Autodesk Inventor part; units mm, degrees
ref_plane "YZ Plane" through (0, 0, 0) normal (1, 0, 0) x (0, 1, 0)
ref_plane "XZ Plane" through (0, 0, 0) normal (0, 1, 0) x (-1, 0, 0)
ref_plane "XY Plane" through (0, 0, 0) normal (0, 0, 1) x (1, 0, 0)
sketch "Sketch1" plane through (0, 0, 0) normal (0, 0, 1) x (1, 0, 0)
  line L0 (-9.6332, 12.3072) -> (10.3668, 12.3072)
  line L1 (10.3668, 12.3072) -> (10.3668, -12.6928)
  line L2 (10.3668, -12.6928) -> (-9.6332, -12.6928)
  line L3 (-9.6332, -12.6928) -> (-9.6332, 12.3072)
  line L4 (-4.3832, -2.6928) -> (5.1168, -2.6928)
  line L5 (5.1168, -2.6928) -> (5.1168, -7.7928)
  line L6 (5.1168, -7.7928) -> (-4.3832, -7.7928)
  line L7 (-4.3832, -7.7928) -> (-4.3832, -2.6928)
  line L8 (-1.0332, -2.6928) -> (-1.0332, -7.7928)
  line L9 (1.7668, -2.6928) -> (1.7668, -7.7928)
  line L10 (-1.0332, -2.6928) -> (-1.0332, 0.3072)
  line L11 (1.7668, -2.6928) -> (1.7668, 0.3072)
  line L12 (-1.0332, 0.3072) -> (-6.6332, 12.3072)
  line L13 (1.7668, 0.3072) -> (7.3668, 12.3072)
  line L14 (-1.0332, -7.7928) -> (-1.0332, -12.6928)
  line L15 (1.7668, -7.7928) -> (1.7668, -12.6928)
  point P0 (0, 0)
  dimension "d0" = 20
  dimension "d1" = 25
  dimension "d2" = 3.35
  dimension "d3" = 3.35
  dimension "d4" = 2.8
  dimension "d5" = 5.1
  dimension "d6" = 5.25
  dimension "d7" = 9.5
  dimension "d9" = 15
  dimension "d10" = 4.9
  dimension "d11" = 3
  dimension "d12" = 3
  dimension "d13" = 3
  dimension "d14" = 3
extrude "Extrusion1" add sketch "Sketch1" along normal blind 3 contours L0 L12 L10 L4 L7 L6 L14 L2 L3 | L0 L1 L2 L15 L6 L5 L4 L11 L13
extrude "Extrusion2" add sketch "Sketch1" against normal blind 5 contours L0 L12 L10 L4 L7 L6 L14 L2 L3 | L0 L13 L11 L4 L10 L12 | L0 L1 L2 L15 L6 L5 L4 L11 L13 | L14 L6 L15 L2 | L4 L9 L6 L8
sketch "Sketch2" plane through (0, 0, -5) normal (0, 0, -1) x (-1, 0, 0)
  line L0 (-1.7668, -2.6928) -> (-1.7668, -7.7928)
  line L1 (-1.7668, -7.7928) -> (-5.1168, -7.7928)
  line L2 (-5.1168, -7.7928) -> (-5.1168, -2.6928)
  line L3 (-5.1168, -2.6928) -> (-1.7668, -2.6928)
  line L4 (1.0332, -7.7928) -> (1.0332, -2.6928)
  line L5 (1.0332, -2.6928) -> (4.3832, -2.6928)
  line L6 (4.3832, -2.6928) -> (4.3832, -7.7928)
  line L7 (4.3832, -7.7928) -> (1.0332, -7.7928)
  line L8 (9.6332, 12.3072) -> (-10.3668, 12.3072)
  line L9 (-10.3668, 12.3072) -> (-10.3668, -12.6928)
  line L10 (-10.3668, -12.6928) -> (9.6332, -12.6928)
  line L11 (9.6332, -12.6928) -> (9.6332, 12.3072)
  line L12 (1.0332, -12.6928) -> (1.0332, -7.7928)
  line L13 (-1.7668, -2.6928) -> (1.0332, -2.6928)
  line L14 (1.0332, -2.6928) -> (1.0332, -7.7928)
  line L15 (1.0332, -7.7928) -> (-1.7668, -7.7928)
  line L16 (-1.7668, -7.7928) -> (-1.7668, -2.6928)
  point P0 (0, 0)
extrude "Extrusion3" cut sketch "Sketch2" against normal blind 3.6 contours L13 L4 L15 L0
chamfer "Chamfer1" distance 12 distance2 3 1 edges at (0.3668, 12.3072, 0) measured on face at (-0.0999, 8.3072, 0)
sketch "Sketch3" plane through (0, 0, 3) normal (0, 0, 1) x (1, 0, 0)
  line L0 (-9.6332, 12.3072) -> (-9.6332, -12.6928)
  line L1 (-9.6332, -12.6928) -> (-1.0332, -12.6928)
  line L2 (-1.0332, -12.6928) -> (-1.0332, -7.7928)
  line L3 (-1.0332, -7.7928) -> (-4.3832, -7.7928)
  line L4 (-4.3832, -7.7928) -> (-4.3832, -2.6928)
  line L5 (-4.3832, -2.6928) -> (-1.0332, -2.6928)
  line L6 (-1.0332, -2.6928) -> (-1.0332, 0.3072)
  line L7 (-1.0332, 0.3072) -> (-6.6332, 12.3072)
  line L8 (-6.6332, 12.3072) -> (-9.6332, 12.3072)
  line L9 (10.3668, -12.6928) -> (10.3668, 12.3072)
  line L10 (10.3668, 12.3072) -> (7.3668, 12.3072)
  line L11 (7.3668, 12.3072) -> (1.7668, 0.3072)
  line L12 (1.7668, 0.3072) -> (1.7668, -2.6928)
  line L13 (1.7668, -2.6928) -> (5.1168, -2.6928)
  line L14 (5.1168, -2.6928) -> (5.1168, -7.7928)
  line L15 (5.1168, -7.7928) -> (1.7668, -7.7928)
  line L16 (1.7668, -7.7928) -> (1.7668, -12.6928)
  line L17 (1.7668, -12.6928) -> (10.3668, -12.6928)
  point P0 (0, 0)
  point P1 (-6.6332, 5.8072)
  point P2 (7.3668, 5.8072)
  point P3 (-6.6332, -9.6928)
  point P4 (7.3668, -9.6928)
  dimension "d24" = 25
  dimension "d25" = 6.5
  dimension "d26" = 3
  dimension "d27" = 4.9
  dimension "d28" = 3
  dimension "d29" = 3
  dimension "d37" = 5.25
  dimension "d38" = 3
  dimension "d39" = 3
hole "Hole1" at (-6.6332, 5.8072, 3) at (7.3668, 5.8072, 3) at (-6.6332, -9.6928, 3) at (7.3668, -9.6928, 3) direction (0, 0, -1) diameter 2.5 end through all
fillet "Fillet1" radius 1.5 2 edges at (-6.6332, 12.3072, 0) (7.3668, 12.3072, 0)
fillet "Fillet2" radius 2 4 edges at (-9.6332, 12.3072, -1) (10.3668, 12.3072, -1) (10.3668, -12.6928, -1) (-9.6332, -12.6928, -1)
equation "\"d3\" = d2"
equation "\"d6\" = -0.5 * d7 + 0.5 * d0"
equation "\"d12\" = d11"
equation "\"d14\" = d13"
properties part number "3DP_PLA_Part_Detector_Bottom_Half" material "ABS Plastic"
The listing builds one solid part. Answer for the finished solid, in the listing's coordinates (mm). A direction names the side the tool comes from. Coordinates: 2 decimals unless noted, no trailing zeros. Write each loop counter-clockwise with the first axis right and the second up, starting at its lowest first coordinate (ties: lowest second). Pieces come first, ordered by that corner, then holes. Notation, with made-up numbers: (53.25, 74) - (81.25, 74) arc R30 ccw to (81.25, 101) - close; hole circle Ø4 at (80, -22.75). An arc over 180 degrees is marked (long way). Answer as CSV lines item,"result".
1. Straight lines are drawn through the part: line 1 (X direction, y = -7.5, z = 1.5); line 2 (Y direction, x = -5.75, z = 2.75); line 3 (X direction, y = 5, z = 1.5). For each, find the intervals that lie inside material, in ascending order. Write a range as [from, to].
Computed values:
line 1,"x = [-9.63, -4.38], [5.12, 10.37]"
line 2,"y = [-12.69, -10.58], [-8.81, 4.92], [6.69, 10.41]"
line 3,"x = [-9.63, -7.59], [-5.68, -3.22], [3.96, 6.41], [8.32, 10.37]"
2. Find section C-C (x = -2.5). Give the vertices of the cut face in (y, z).
Computed values:
outline,"(-12.69, -5) - (-7.79, -5) - (-7.79, 3) - (-12.69, 3) - close; (-2.69, -5) - (12.31, -5) - (12.31, -3) - (3.45, -0.79) - (3.45, 3) - (-2.69, 3) - close"
3. A tool of negligible diameter and unlimited length cuts with its end or side. For faces 1 (the flat face through (-1.033, -1, 1)), 2 (the cylindrical face through (7.53, 12.08, 0.04)), 3 (the flat face through (-4.383, -5, -1)), from which of +Z, -Z, +X, -X, +Y, -Y can it reach the whole face along a straight path? Write none if from no direction.
Computed values:
face 1,"+Z, +Y, -Y"
face 2,"+Z, +Y"
face 3,"+Z, -Z"
4. Given P1, Ø2, axis at x = 0, y = -4.5, coming from the -Z side, flat-ended and moving along its own axis, determine where the tip first touches the part or whether it passes through.
Computed values:
P1,"stops at z = -1.4"
5. Find section D-D (z = -2). Give the vertices of the cut face in (x, y), plus the area to 3 significant figures.
Computed values:
outline,"(-9.63, -10.69) arc R2 ccw to (-7.63, -12.69) - (8.37, -12.69) arc R2 ccw to (10.37, -10.69) - (10.37, 10.31) arc R2 ccw to (8.37, 12.31) - (8.32, 12.31) arc R1.5 ccw to (6.96, 11.44) - (5.5, 8.31) - (-4.77, 8.31) - (-6.23, 11.44) arc R1.5 ccw to (-7.59, 12.31) - (-7.63, 12.31) arc R2 ccw to (-9.63, 10.31) - close; hole circle Ø2.5 at (-6.63, -9.69); hole circle Ø2.5 at (-6.63, 5.81); hole (-4.38, -7.79) - (5.12, -7.79) - (5.12, -2.69) - (-4.38, -2.69) - close; hole circle Ø2.5 at (7.37, -9.69); hole circle Ø2.5 at (7.37, 5.81)"
area,"380 mm²"
6. Find section B-B (y = -3.75). Give the vertices of the cut face in (x, z), plus the area to 3 significant figures.
Computed values:
outline,"(-9.63, -5) - (-4.38, -5) - (-4.38, 3) - (-9.63, 3) - close; (-1.03, -1.4) - (1.77, -1.4) - (1.77, 0) - (-1.03, 0) - close; (5.12, -5) - (10.37, -5) - (10.37, 3) - (5.12, 3) - close"
area,"87.9 mm²"
7. Find section A-A (z = 1). Give the vertices of the cut face in (x, y).
Computed values:
outline,"(-9.63, -10.69) arc R2 ccw to (-7.63, -12.69) - (-1.03, -12.69) - (-1.03, -7.79) - (-4.38, -7.79) - (-4.38, -2.69) - (-1.03, -2.69) - (-1.03, 0.31) - (-6.23, 11.44) arc R1.5 ccw to (-7.59, 12.31) - (-7.63, 12.31) arc R2 ccw to (-9.63, 10.31) - close; (1.77, -12.69) - (8.37, -12.69) arc R2 ccw to (10.37, -10.69) - (10.37, 10.31) arc R2 ccw to (8.37, 12.31) - (8.32, 12.31) arc R1.5 ccw to (6.96, 11.44) - (1.77, 0.31) - (1.77, -2.69) - (5.12, -2.69) - (5.12, -7.79) - (1.77, -7.79) - close; hole circle Ø2.5 at (-6.63, -9.69); hole circle Ø2.5 at (-6.63, 5.81); hole circle Ø2.5 at (7.37, -9.69); hole circle Ø2.5 at (7.37, 5.81)"
8. Determine the mould class of faces 4 (the flat face through (0, 12.307, -4)), 5 (the flat face through (1.767, -10, 1)), 6 (the flat face through (10.367, 0, -1)), 7 (the cylindrical face through (-9.03, 11.74, -0.94)) for opening direction X: +X half, -X half, draft (parallel to the pull), parting line (faces both ways), or undercut.
Computed values:
face 4,"draft"
face 5,"undercut"
face 6,"+X half"
face 7,"-X half"
